Source: CAD feature listing. Evaluate the final solid. Frame: model axes, mm. A direction names the side the tool comes from. Give positions to 0.01 mm unless a question says otherwise; leave off trailing zeros. Loops run counter-clockwise (first coordinate to the right, second up) from the corner with the lowest first, then second, coordinate; pieces in that order, holes last. Notation, with made-up numbers: (8.5, -3) -> (67.5, -3) arc R33 cw to (67.5, 32) -> close; hole circle Ø9 at (-14.75, -37.75). An arc over 180 degrees is marked (long way). Return JSON: item names as keys, results as strings. Group by question number.
(1) Cut plane D-D on x = 58. Return loops of the section in (y, z).
(2) Draft query along Z for faces 4 (the face through (9.86, 11.5, -14.77)), 5 (the face through (9.86, 11.5, 5.23)), 6 (the face through (24.79, 34.168, -7.587)), 7 (the face through (10, 15, 15)). Return one class per face: released by +Z, released by -Z, zero draft, split by the parting line, or undercut.
(3) Pin query (flat end, axial travel): pin 1 (1 mm diameter, centred on x = 18, z = -25, fed in from +Y) (3 decimals); pin 2 (5 mm diameter, centred on x = 30, y = -27.5, fed in from +Z); pin 3 (8 mm diameter, centred on x = 34, y = 17.5, fed in from -Z). Return the tip coordinate at first contact, or that it passes through.
(4) Cut plane B-B on x = 7. Return loops of the section in (y, z).
(5) Cut plane C-C on y = -13. Return loops of the section in (x, z).
(6) Ray query, line 1 (X direction, y = -27, z = -21); line 2 (X direction, y = 8.5, z = -17.5); line 3 (Y direction, x = 7.75, z = -10). Return the intervals inside material, ascending. Write a range as from..to.
(7) Access query for faces 1 (the face through (100, 0, 0)), 2 (the face through (4.93, -0.88, -19.98)), 3 (the face through (69.58, -12.65, 8.06)). Directions: +Z, -Z, +X, -X, +Y, -Y. A direction counts if a zero-diameter tool reaches every point of the face in a straight line with its end or side. Return the directions, or none.
(8) Cut plane A-A on z = 0. Return loops of the section in (x, y).
```python
from build123d import *

# Parameters (mm, degrees)
SKETCH_2_R          = 5
CUT_EXTRUDE_1_DEPTH = 20
SKETCH_3_R          = 5
CUT_EXTRUDE_2_DEPTH = 20


with BuildPart() as part:
    # Эскиз1 → Повернуть1 (revolve)
    with BuildSketch(Plane.XY, mode=Mode.PRIVATE) as revolve_1_sk:
        Polygon((0, 0), (100, 0), (100, 15), (40, 15), (40, 35), (10, 35), (10, 20), (0, 20), align=None)
    revolve(revolve_1_sk.sketch.rotate(Axis((0, 0, 0), (1, 0, 0)), 90), axis=Axis((0, 0, 0), (1, 0, 0)))

    # Эскиз2 → Вырез-Вытянуть1 (cut)
    with BuildSketch(Plane(origin=(0, 0, 0), x_dir=(0, 0, -1), z_dir=(1, 0, 0))):
        with Locations((10, 10)):
            Circle(SKETCH_2_R)
    extrude(amount=CUT_EXTRUDE_1_DEPTH, mode=Mode.SUBTRACT)

    # Эскиз3 → Вырез-Вытянуть2 (cut)
    with BuildSketch(Plane(origin=(0, 0, 0), x_dir=(0, 0, -1), z_dir=(1, 0, 0))):
        with Locations((-10, 10)):
            Circle(SKETCH_3_R)
    extrude(amount=CUT_EXTRUDE_2_DEPTH, mode=Mode.SUBTRACT)


solid = part.part
```
Answers:
{
 "1": {"outline": "circle Ø30 at (0, 0)"},
 "2": {"face 4": "undercut", "face 5": "undercut", "face 6": "split by the parting line", "face 7": "zero draft"},
 "3": {"pin 1": "y = 24.995", "pin 2": "z = 24.49", "pin 3": "z = -32.29"},
 "4": {"outline": "circle Ø40 at (0, 0); hole circle Ø10 at (10, -10); hole circle Ø10 at (10, 10)"},
 "5": {"outline": "(0, -15.2) -> (10, -15.2) -> (10, -32.5) -> (40, -32.5) -> (40, -7.48) -> (100, -7.48) -> (100, 7.48) -> (40, 7.48) -> (40, 32.5) -> (10, 32.5) -> (10, 15.2) -> (0, 15.2) -> close"},
 "6": {"line 1": "10..40", "line 2": "0..40", "line 3": "-17.32..5, 15..17.32"},
 "7": {"face 1": "+Z, -Z, +X, +Y, -Y", "face 2": "-X", "face 3": "+X"},
 "8": {"outline": "(0, -20) -> (10, -20) -> (10, -35) -> (40, -35) -> (40, -15) -> (100, -15) -> (100, 15) -> (40, 15) -> (40, 35) -> (10, 35) -> (10, 20) -> (0, 20) -> close"}
}
